The model under review builds one solid part; all positions refer to its coordinate system, in mm. Face numbers are marked on the shaded views. Coordinates: 2 decimals unless noted, no trailing zeros. Write each loop counter-clockwise with the first axis right and the second up, starting at its lowest first coordinate (ties: lowest second). Pieces come first, ordered by that corner, then holes. Notation, with made-up numbers: (-4, 38) - (54, 38) arc R33 cw to (54, 75) - close; hole circle Ø6 at (-16, -17). An arc over 180 degrees is marked (long way). Return JSON: item names as keys, results as strings. Group by question number.
(1) We need section D-D on x = -8.5. State the section outline as (y, z) points.
(2) For pin 1 Ø1.5 at (y, z) = (5.5, 3.5) entering from +X; pin 2 Ø1.5 at (y, z) = (-1.5, 3.5) entering from -X; pin 3 Ø2 at (x, y) = (17, 3.5) entering from +Z, all flat-tipped, find the tip position at first contact; note any pin that passes through.
(3) We need section A-A on x = 0. State the section outline as (y, z) points, then the cut area to 3 significant figures.
(4) We need section C-C on y = -7.5. State the section outline as (x, z) points, then the cut area to 3 significant figures.
(5) Draft analysis for pull direction Y (two halves, no side actions). For the marked faces 1, 2 and 3, state which applies: released by +Y, released by -Y, zero draft, split by the parting line, or undercut.
(6) We need section B-B on y = 7.5. State the section outline as (x, z) points, then the cut area to 3 significant figures.
(7) To check wall thickness, follow L1, parallel to Y at x = 0, z = 0.7; L2, parallel to Y at x = 1, z = 1.9; L3, parallel to Z at x = -5.5, y = -13. State the ranges of each line that lie inside material, in increasing order. Write a range as from..to.
```python
from build123d import *

# Parameters (mm, degrees)
SKETCH_1_R      = 21.5
SKETCH_1_R_2    = 10.6
SKETCH_1_R_3    = 1.5
EXTRUDE_1_DEPTH = 3
SKETCH_2_R      = 1.5
EXTRUDE_2_DEPTH = 1.4


with BuildPart() as part:
    # 草圖1 → 填料-伸長1 (new body)
    with BuildSketch(Plane.XY):
        Circle(SKETCH_1_R)
        Circle(SKETCH_1_R_2, mode=Mode.SUBTRACT)
        with Locations((0, 15)):
            Circle(SKETCH_1_R_3, mode=Mode.SUBTRACT)
        with Locations((12.990381057, -7.5)):
            Circle(SKETCH_1_R_3, mode=Mode.SUBTRACT)
        with Locations((-12.990381057, -7.5)):
            Circle(SKETCH_1_R_3, mode=Mode.SUBTRACT)
    extrude(amount=EXTRUDE_1_DEPTH)

    # 草圖2 → 填料-伸長2 (add)
    with BuildSketch(Plane.XY.offset(3)):
        with Locations((12.990381057, 7.5)):
            Circle(SKETCH_2_R)
        with Locations((-12.990381057, 7.5)):
            Circle(SKETCH_2_R)
        with Locations((0, -15)):
            Circle(SKETCH_2_R)
    extrude(amount=EXTRUDE_2_DEPTH)


solid = part.part
```
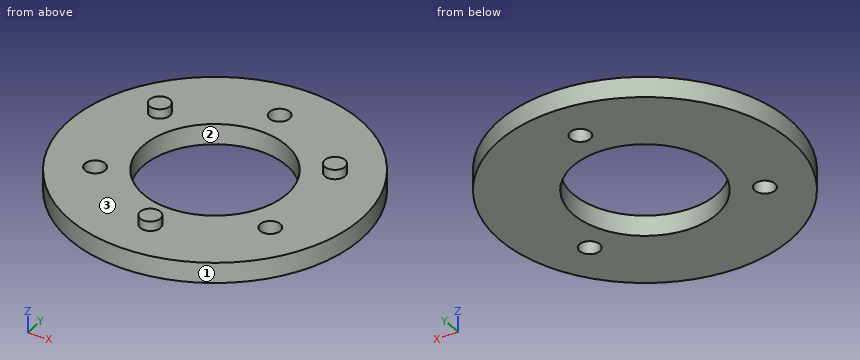
Ans:
{
 "1": {"outline": "(-19.75, 0) - (-6.33, 0) - (-6.33, 3) - (-19.75, 3) - close; (6.33, 0) - (19.75, 0) - (19.75, 3) - (6.33, 3) - close"},
 "2": {"pin 1": "x = 20.92", "pin 2": "x = -21.48", "pin 3": "z = 3"},
 "3": {"outline": "(-21.5, 0) - (-10.6, 0) - (-10.6, 3) - (-13.5, 3) - (-13.5, 4.4) - (-16.5, 4.4) - (-16.5, 3) - (-21.5, 3) - close; (10.6, 0) - (13.5, 0) - (13.5, 3) - (10.6, 3) - close; (16.5, 0) - (21.5, 0) - (21.5, 3) - (16.5, 3) - close", "area": "60.6 mm²"},
 "4": {"outline": "(-20.15, 0) - (-14.49, 0) - (-14.49, 3) - (-20.15, 3) - close; (-11.49, 0) - (-7.49, 0) - (-7.49, 3) - (-11.49, 3) - close; (7.49, 0) - (11.49, 0) - (11.49, 3) - (7.49, 3) - close; (14.49, 0) - (20.15, 0) - (20.15, 3) - (14.49, 3) - close", "area": "58.0 mm²"},
 "5": {"face 1": "split by the parting line", "face 2": "undercut", "face 3": "zero draft"},
 "6": {"outline": "(-20.15, 0) - (-7.49, 0) - (-7.49, 3) - (-11.49, 3) - (-11.49, 4.4) - (-14.49, 4.4) - (-14.49, 3) - (-20.15, 3) - close; (7.49, 0) - (20.15, 0) - (20.15, 3) - (14.49, 3) - (14.49, 4.4) - (11.49, 4.4) - (11.49, 3) - (7.49, 3) - close", "area": "84.4 mm²"},
 "7": {"L1": "-21.5..-10.6, 10.6..13.5, 16.5..21.5", "L2": "-21.48..-10.55, 10.55..13.88, 16.12..21.48", "L3": "0..3"}
}
